Autodesk Fusion 360 part; units mm, degrees
sketch "Sketch1" plane through (0, 0, 0) normal (0, 1, 0) x (1, 0, 0)
  circle A0 centre (0, 0) radius 25
  line L0 (0, 0) -> (0, -50) construction
  line L1 (0, -45) -> (-5, -45)
  line L2 (-5, -45) -> (-5, -38.6782)
  line L3 (5, -45) -> (5, -38.6782)
  line L4 (0, -45) -> (5, -45)
  line L5 (12.6014, -43.488) -> (10.1821, -37.6474)
  line L6 (17.2208, -41.5746) -> (12.6014, -43.488)
  line L7 (17.2208, -41.5746) -> (21.8402, -39.6612)
  line L8 (21.8402, -39.6612) -> (19.4209, -33.8205)
  line L9 (28.2843, -35.3553) -> (23.8141, -30.8851)
  line L10 (31.8198, -31.8198) -> (28.2843, -35.3553)
  line L11 (31.8198, -31.8198) -> (35.3553, -28.2843)
  line L12 (35.3553, -28.2843) -> (30.8851, -23.8141)
  line L13 (39.6612, -21.8402) -> (33.8205, -19.4209)
  line L14 (41.5746, -17.2208) -> (39.6612, -21.8402)
  line L15 (41.5746, -17.2208) -> (43.488, -12.6014)
  line L16 (43.488, -12.6014) -> (37.6474, -10.1821)
  line L17 (45, -5) -> (38.6782, -5)
  line L18 (45, 0) -> (45, -5)
  line L19 (45, 0) -> (45, 5)
  line L20 (45, 5) -> (38.6782, 5)
  line L21 (43.488, 12.6014) -> (37.6474, 10.1821)
  line L22 (41.5746, 17.2208) -> (43.488, 12.6014)
  line L23 (41.5746, 17.2208) -> (39.6612, 21.8402)
  line L24 (39.6612, 21.8402) -> (33.8205, 19.4209)
  line L25 (35.3553, 28.2843) -> (30.8851, 23.8141)
  line L26 (31.8198, 31.8198) -> (35.3553, 28.2843)
  line L27 (31.8198, 31.8198) -> (28.2843, 35.3553)
  line L28 (28.2843, 35.3553) -> (23.8141, 30.8851)
  line L29 (21.8402, 39.6612) -> (19.4209, 33.8205)
  line L30 (17.2208, 41.5746) -> (21.8402, 39.6612)
  line L31 (17.2208, 41.5746) -> (12.6014, 43.488)
  line L32 (12.6014, 43.488) -> (10.1821, 37.6474)
  line L33 (5, 45) -> (5, 38.6782)
  line L34 (0, 45) -> (5, 45)
  line L35 (0, 45) -> (-5, 45)
  line L36 (-5, 45) -> (-5, 38.6782)
  line L37 (-12.6014, 43.488) -> (-10.1821, 37.6474)
  line L38 (-17.2208, 41.5746) -> (-12.6014, 43.488)
  line L39 (-17.2208, 41.5746) -> (-21.8402, 39.6612)
  line L40 (-21.8402, 39.6612) -> (-19.4209, 33.8205)
  line L41 (-28.2843, 35.3553) -> (-23.8141, 30.8851)
  line L42 (-31.8198, 31.8198) -> (-28.2843, 35.3553)
  line L43 (-31.8198, 31.8198) -> (-35.3553, 28.2843)
  line L44 (-35.3553, 28.2843) -> (-30.8851, 23.8141)
  line L45 (-39.6612, 21.8402) -> (-33.8205, 19.4209)
  line L46 (-41.5746, 17.2208) -> (-39.6612, 21.8402)
  line L47 (-41.5746, 17.2208) -> (-43.488, 12.6014)
  line L48 (-43.488, 12.6014) -> (-37.6474, 10.1821)
  line L49 (-45, 5) -> (-38.6782, 5)
  line L50 (-45, 0) -> (-45, 5)
  line L51 (-45, 0) -> (-45, -5)
  line L52 (-45, -5) -> (-38.6782, -5)
  line L53 (-43.488, -12.6014) -> (-37.6474, -10.1821)
  line L54 (-41.5746, -17.2208) -> (-43.488, -12.6014)
  line L55 (-41.5746, -17.2208) -> (-39.6612, -21.8402)
  line L56 (-39.6612, -21.8402) -> (-33.8205, -19.4209)
  line L57 (-35.3553, -28.2843) -> (-30.8851, -23.8141)
  line L58 (-31.8198, -31.8198) -> (-35.3553, -28.2843)
  line L59 (-31.8198, -31.8198) -> (-28.2843, -35.3553)
  line L60 (-28.2843, -35.3553) -> (-23.8141, -30.8851)
  line L61 (-21.8402, -39.6612) -> (-19.4209, -33.8205)
  line L62 (-17.2208, -41.5746) -> (-21.8402, -39.6612)
  line L63 (-17.2208, -41.5746) -> (-12.6014, -43.488)
  line L64 (-12.6014, -43.488) -> (-10.1821, -37.6474)
  arc A1 (-10.1821, -37.6474) -> (-5, -38.6782) centre (0, 0) ccw
  arc A2 (-23.8141, -30.8851) -> (-19.4209, -33.8205) centre (0, 0) ccw
  arc A3 (-33.8205, -19.4209) -> (-30.8851, -23.8141) centre (0, 0) ccw
  arc A4 (-38.6782, -5) -> (-37.6474, -10.1821) centre (0, 0) ccw
  arc A5 (-37.6474, 10.1821) -> (-38.6782, 5) centre (0, 0) ccw
  arc A6 (-30.8851, 23.8141) -> (-33.8205, 19.4209) centre (0, 0) ccw
  arc A7 (-19.4209, 33.8205) -> (-23.8141, 30.8851) centre (0, 0) ccw
  arc A8 (-5, 38.6782) -> (-10.1821, 37.6474) centre (0, 0) ccw
  arc A9 (10.1821, 37.6474) -> (5, 38.6782) centre (0, 0) ccw
  arc A10 (23.8141, 30.8851) -> (19.4209, 33.8205) centre (0, 0) ccw
  arc A11 (38.6782, 5) -> (37.6474, 10.1821) centre (0, 0) ccw
  arc A12 (33.8205, 19.4209) -> (30.8851, 23.8141) centre (0, 0) ccw
  arc A13 (37.6474, -10.1821) -> (38.6782, -5) centre (0, 0) ccw
  arc A14 (30.8851, -23.8141) -> (33.8205, -19.4209) centre (0, 0) ccw
  arc A15 (5, -38.6782) -> (10.1821, -37.6474) centre (0, 0) ccw
  arc A16 (19.4209, -33.8205) -> (23.8141, -30.8851) centre (0, 0) ccw
  dimension "d1" = 50
  dimension "d2" = 78
  dimension "d4" = 5
extrude "Extrude1" add sketch "Sketch1" along normal blind 10
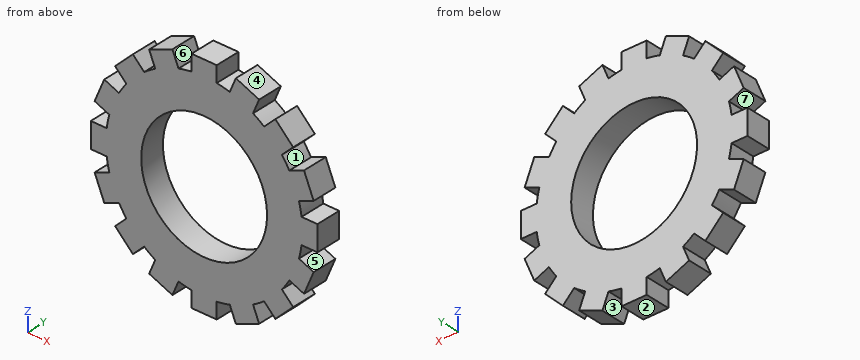
Source: CAD feature listing. Evaluate the final solid. Frame: model axes, mm. Face numbers are marked on the shaded views. A direction names the side the tool comes from. Give positions to 0.01 mm unless a question says otherwise; leave off trailing zeros. Loops run counter-clockwise (first coordinate to the right, second up) from the corner with the lowest first, then second, coordinate; pieces in that order, holes last. Notation, with made-up numbers: (87, 21) -> (130, 21) arc R34 ccw to (130, 56) -> close; hole circle Ø1 at (65, -7.5). An arc over 180 degrees is marked (long way). Put each result on its own line as item: value. Start each with the question number.
1) Cut plane B-B (x = 0). Return loops of the section in (y, z), then the cut area to 3 significant figures.
2) Reachability of the marked faces 5, 6 and 7 from +Z, -Z, +X, -X, +Y, -Y: full face, straight path, thin tool, end or side. Return the list, or none.
3) Draft query along X for the marked faces 1, 2, 3 and 4. Return one class per face: released by +X, released by -X, zero draft, split by the parting line, or undercut.
4) Material intervals for probe 1 along Z at (x, y) = (0, 7.25); probe 2 along X at (y, z) = (7.5, -21), sorted ascending.
5) Cut plane A-A (z = 0). Return loops of the section in (x, y), then the cut area to 3 significant figures.
6) Contact query for flat-ended pins moving along their axis: P1, Ø3, axis at y = 7, z = -22.5, coming from the +X side; P2, Ø4, axis at x = 32.5, y = 7.5, coming from the -Z side; P3, Ø1, axis at x = -13, y = 1.5, coming from the +Z side. Output: stop coordinate, or through.
Results are:
1. outline: (0, -45) -> (10, -45) -> (10, -25) -> (0, -25) -> close; (0, 25) -> (10, 25) -> (10, 45) -> (0, 45) -> close
1. area: 400 mm2
2. face 5: +X, +Y, -Y
2. face 6: +Z, +Y, -Y
2. face 7: -X, +Y, -Y
3. face 1: undercut
3. face 2: zero draft
3. face 3: undercut
3. face 4: released by +X
4. probe 1: z = -45 to -25, 25 to 45
4. probe 2: x = -40.01 to -37.63, -32.86 to -13.56, 13.56 to 32.86, 37.63 to 40.01
5. outline: (-45, 0) -> (-25, 0) -> (-25, 10) -> (-45, 10) -> close; (25, 0) -> (45, 0) -> (45, 10) -> (25, 10) -> close
5. area: 400 mm2
6. P1: stops at x = 40.01
6. P2: stops at z = -33.14
6. P3: stops at z = 43.49
